CAD build for the part. Positions are in the model's coordinates, mm. Round coordinates to 2 decimals unless told otherwise and drop trailing zeros. Loops run counter-clockwise (first coordinate to the right, second up) from the corner with the lowest first, then second, coordinate; pieces in that order, holes last.
from build123d import *

# Parameters (mm, degrees)
SKETCH_1_R             = 60
SM_BASE_FLANGE_1_DEPTH = 2
CUT_EXTRUDE_2_REACH    = 86.876
SKETCH_7_R             = 44
CUT_EXTRUDE_1_REACH    = 86.876
SKETCH_6_R             = 1.5


# Sheet-metal steps are written as plain solids
with BuildPart() as part:
    # Sketch 1 → 基体-法兰1 (new body)
    with BuildSketch(Plane(origin=(0, 0, 0), x_dir=(1, 0, 0), z_dir=(0, 1, 0))):
        with Locations(Location((0, 0, 0), (0, 0, 270))):
            Circle(SKETCH_1_R)
    extrude(amount=-SM_BASE_FLANGE_1_DEPTH)

    # 草图7 → 切除-拉伸2 (cut, up to next)
    with BuildSketch(Plane(origin=(0, 0, 0), x_dir=(1, 0, 0), z_dir=(0, 1, 0)), mode=Mode.PRIVATE) as cut_extrude_2_sk1:
        with Locations(Location((0, 0, 0), (0, 0, 270))):
            Circle(SKETCH_7_R)
    cut_extrude_2_tool1 = extrude(cut_extrude_2_sk1.sketch, amount=-CUT_EXTRUDE_2_REACH, mode=Mode.PRIVATE) & part.part
    add(cut_extrude_2_tool1.solids().sort_by_distance((0, 0, 0))[0], mode=Mode.SUBTRACT)

    # 草图6 → 切除-拉伸1 (cut, up to next)
    with BuildSketch(Plane(origin=(0, 0, 0), x_dir=(1, 0, 0), z_dir=(0, 1, 0)), mode=Mode.PRIVATE) as cut_extrude_1_sk1:
        with Locations(Location((-36.769552622, -36.769552622, 0), (0, 0, 270))):
            Circle(SKETCH_6_R)
    cut_extrude_1_tool1 = extrude(cut_extrude_1_sk1.sketch, amount=-CUT_EXTRUDE_1_REACH, mode=Mode.PRIVATE) & part.part
    # 草图6 → 切除-拉伸1 (cut, up to next)
    with BuildSketch(Plane(origin=(0, 0, 0), x_dir=(1, 0, 0), z_dir=(0, 1, 0)), mode=Mode.PRIVATE) as cut_extrude_1_sk2:
        with Locations(Location((-36.769552622, 36.769552622, 0), (0, 0, 270))):
            Circle(SKETCH_6_R)
    cut_extrude_1_tool2 = extrude(cut_extrude_1_sk2.sketch, amount=-CUT_EXTRUDE_1_REACH, mode=Mode.PRIVATE) & part.part
    # 草图6 → 切除-拉伸1 (cut, up to next)
    with BuildSketch(Plane(origin=(0, 0, 0), x_dir=(1, 0, 0), z_dir=(0, 1, 0)), mode=Mode.PRIVATE) as cut_extrude_1_sk3:
        with Locations(Location((36.769552622, 36.769552622, 0), (0, 0, 270))):
            Circle(SKETCH_6_R)
    cut_extrude_1_tool3 = extrude(cut_extrude_1_sk3.sketch, amount=-CUT_EXTRUDE_1_REACH, mode=Mode.PRIVATE) & part.part
    # 草图6 → 切除-拉伸1 (cut, up to next)
    with BuildSketch(Plane(origin=(0, 0, 0), x_dir=(1, 0, 0), z_dir=(0, 1, 0)), mode=Mode.PRIVATE) as cut_extrude_1_sk4:
        with Locations(Location((36.769552622, -36.769552622, 0), (0, 0, 270))):
            Circle(SKETCH_6_R)
    cut_extrude_1_tool4 = extrude(cut_extrude_1_sk4.sketch, amount=-CUT_EXTRUDE_1_REACH, mode=Mode.PRIVATE) & part.part
    add(cut_extrude_1_tool1.solids().sort_by_distance((-36.769553, 0, 36.769553))[0], mode=Mode.SUBTRACT)
    add(cut_extrude_1_tool2.solids().sort_by_distance((-36.769553, 0, -36.769553))[0], mode=Mode.SUBTRACT)
    add(cut_extrude_1_tool3.solids().sort_by_distance((36.769553, 0, -36.769553))[0], mode=Mode.SUBTRACT)
    add(cut_extrude_1_tool4.solids().sort_by_distance((36.769553, 0, 36.769553))[0], mode=Mode.SUBTRACT)


solid = part.part
Item 1: Wall check: L1, parallel to Z at x = 38, y = -0.35; L2, parallel to Z at x = 1.5, y = -1.4; L3, parallel to Z at x = -26, y = -1. Give the ranges that are in metal, low to high.
Verdict:
L1: z = -46.43 to -37.63, -35.91 to -22.18, 22.18 to 35.91, 37.63 to 46.43
L2: z = -59.98 to -43.97, 43.97 to 59.98
L3: z = -54.07 to -35.5, 35.5 to 54.07
Item 2: Cut at B-B (z = 0). List the corners of the cut face in (x, y), plus the area to 3 significant figures.
Verdict:
outline: (-60, -2) - (-44, -2) - (-44, 0) - (-60, 0) - close; (44, -2) - (60, -2) - (60, 0) - (44, 0) - close
area: 64.0 mm2
Item 3: Flat gauge pin, fed straight in: P1, Ø1, axis at y = -1.5, z = 2.5, coming from the -X side. Where does the tip first touch, or does it go through?
Verdict:
P1: stops at x = -59.97
Item 4: Mould opens along X. For faces 1 (the cylindrical face through (2.64, -0.99, -59.94)), 2 (the cylindrical face through (-37.68, -0.99, -37.96)), 3 (the cylindrical face through (35.857, -0.986, 35.579)), 4 (the flat face through (40.3, 0, -18.1)) say: released by +X, released by -X, zero draft, split by the parting line, or undercut.
Verdict:
face 1: split by the parting line
face 2: undercut
face 3: undercut
face 4: zero draft
Item 5: Cut at C-C (x = -51). List the corners of the cut face in (y, z).
Verdict:
outline: (-2, -31.61) - (0, -31.61) - (0, 31.61) - (-2, 31.61) - close
Item 6: Cut at A-A (x = 0). List the corners of the cut face in (y, z), plus the area to 3 significant figures.
Verdict:
outline: (-2, -60) - (0, -60) - (0, -44) - (-2, -44) - close; (-2, 44) - (0, 44) - (0, 60) - (-2, 60) - close
area: 64.0 mm2
